Study the drawing (mm; zero at the part's minimum x, y, z) and answer. A direction names the side the tool comes from. Coordinates: 2 decimals unless noted, no trailing zeros. Write each loop counter-clockwise with the first axis right and the second up, starting at its lowest first coordinate (ties: lowest second). Pieces come first, ordered by that corner, then holes. Notation, with made-up numbers: (65, 48) - (111, 48) arc R19 ccw to (111, 68) - close; hole circle Ø1 at (-15.75, 59.25). An arc over 180 degrees is marked (long way). One line per item, written item: value.
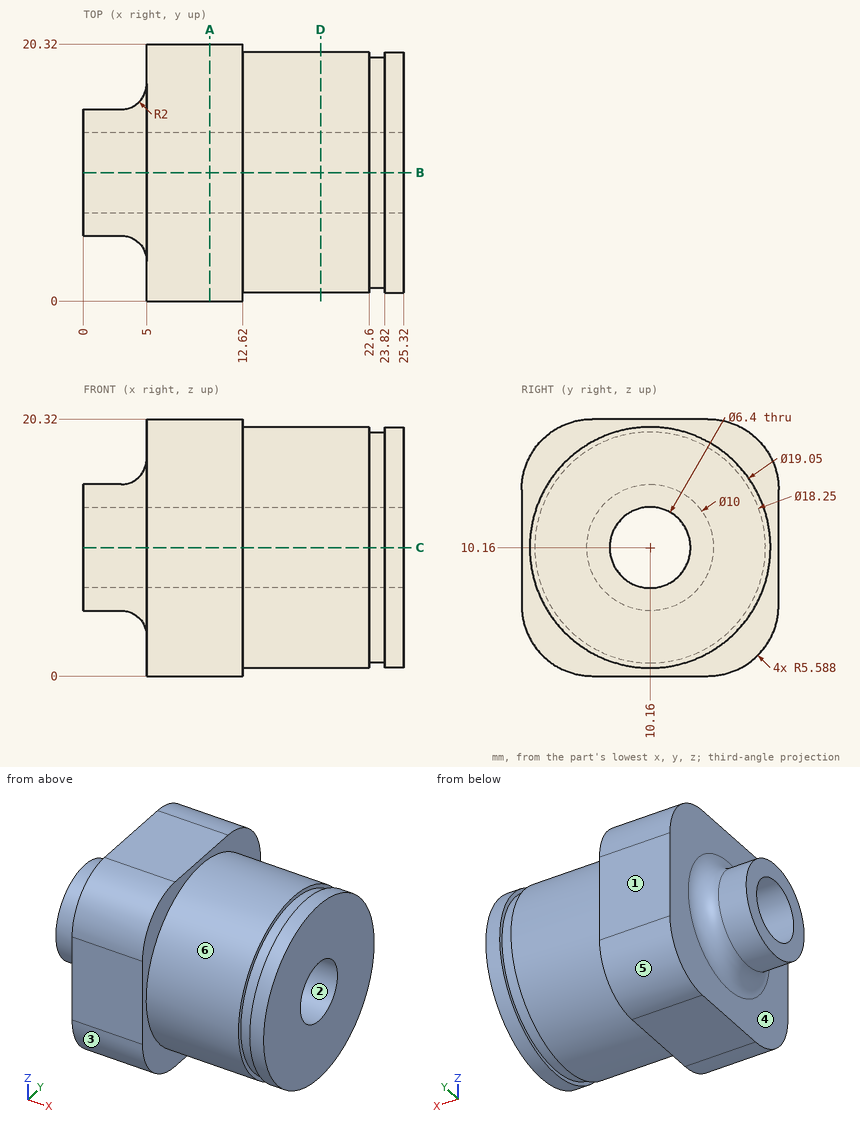
Item 1: Given pin 1 (8 mm diameter, centred on x = 19.5, z = 4, fed in from -Y); pin 2 (8 mm diameter, centred on x = 20, y = 4.5, fed in from -Z), each flat-ended and moving along its own axis, determine where each tip first touches the part or whether it passes through.
Evaluation:
pin 1: stops at y = 0.88
pin 2: stops at z = 0.78
Item 2: Consider probe 1 along Y at (x, z) = (9.75, 10.16); probe 2 along X at (y, z) = (1.75, 10); probe 3 along X at (y, z) = (5.5, 19). Determine where each line is inside the solid, lowest interval first.
Evaluation:
probe 1: y = 0 to 6.96, 13.36 to 20.32
probe 2: x = 5 to 25.32
probe 3: x = 5 to 12.62
Item 3: Section D-D, the plane x = 18.75 is taken. Determine the outline of the cut face in (y, z) (3 decimals).
Evaluation:
outline: circle Ø19.05 at (10.16, 10.16); hole circle Ø6.4 at (10.16, 10.16)
Item 4: Section B-B, the plane y = 10.16 is taken. Determine the outline of the cut face in (x, z) (3 decimals).
Evaluation:
outline: (0, 5.16) - (3, 5.16) arc R2 cw to (5, 3.16) - (5, 0) - (12.62, 0) - (12.62, 0.635) - (22.6, 0.635) - (22.6, 1.035) - (23.82, 1.035) - (23.82, 0.635) - (25.32, 0.635) - (25.32, 6.96) - (0, 6.96) - close; (0, 13.36) - (25.32, 13.36) - (25.32, 19.685) - (23.82, 19.685) - (23.82, 19.285) - (22.6, 19.285) - (22.6, 19.685) - (12.62, 19.685) - (12.62, 20.32) - (5, 20.32) - (5, 17.16) arc R2 cw to (3, 15.16) - (0, 15.16) - close
Item 5: Determine the mould class of the marked faces 1, 2 and 3 for opening direction Y: +Y half, -Y half, draft (parallel to the pull), parting line (faces both ways), or undercut.
Evaluation:
face 1: +Y half
face 2: undercut
face 3: -Y half
Item 6: Which of the six approach directions +Z, -Z, +X, -X, +Y, -Y give full straight-line access (tool end or side, diameter ignored) to the marked faces 4, 5 and 6?
Evaluation:
face 4: -X
face 5: -Z, +X, -X, +Y
face 6: +X
Item 7: Section A-A, the plane x = 10 is taken. Determine the outline of the cut face in (y, z).
Evaluation:
outline: (0, 5.59) arc R5.59 ccw to (5.59, 0) - (14.73, 0) arc R5.59 ccw to (20.32, 5.59) - (20.32, 14.73) arc R5.59 ccw to (14.73, 20.32) - (5.59, 20.32) arc R5.59 ccw to (0, 14.73) - close; hole circle Ø6.4 at (10.16, 10.16)
